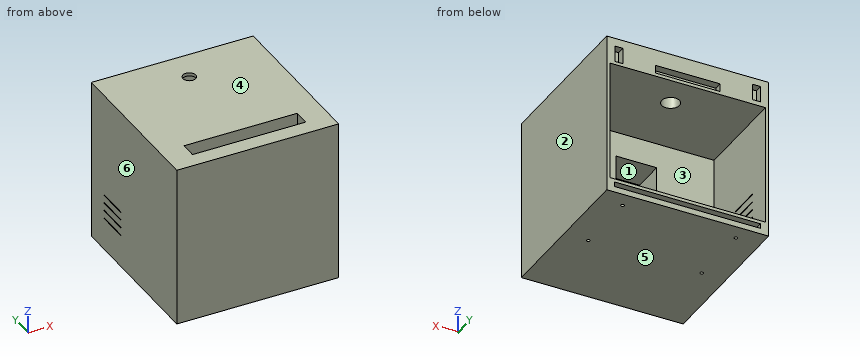
from build123d import *

# Parameters (mm, degrees)
SKETCH1_W           = 100
SKETCH1_H           = 100
BOSS_EXTRUDE1_DEPTH = 100
SKETCH2_W           = 90
SKETCH2_H           = 70
CUT_EXTRUDE1_DEPTH  = 50
SKETCH3_W           = 25
SKETCH3_H           = 25
CUT_EXTRUDE2_DEPTH  = 30
SKETCH4_W           = 70
SKETCH4_H           = 10
CUT_EXTRUDE3_DEPTH  = 70
SKETCH9_W           = 0.5
SKETCH9_H           = 20
CUT_EXTRUDE7_DEPTH  = 10
SKETCH15_W          = 40
SKETCH15_H          = 5
CUT_EXTRUDE8_DEPTH  = 5
SKETCH16_W          = 5
SKETCH16_H          = 10
CUT_EXTRUDE9_DEPTH  = 5
SKETCH17_W          = 5
SKETCH17_H          = 10
CUT_EXTRUDE10_DEPTH = 5
SKETCH20_W          = 70
SKETCH20_H          = 10
CUT_EXTRUDE11_DEPTH = 20
SKETCH21_W          = 90
SKETCH21_H          = 3
CUT_EXTRUDE12_DEPTH = 5
SKETCH23_W          = 90
SKETCH23_H          = 70
CUT_EXTRUDE14_DEPTH = 10
SKETCH26_R          = 1
CUT_EXTRUDE16_DEPTH = 10
SKETCH29_R          = 4
CUT_EXTRUDE20_DEPTH = 11
CUT_EXTRUDE21_START = -2
SKETCH30_R          = 5.5
CUT_EXTRUDE21_DEPTH = 20
SKETCH31_W          = 96
SKETCH31_H          = 74.5
CUT_EXTRUDE22_DEPTH = 60


with BuildPart() as part:
    # Sketch1 → Boss-Extrude1 (new body)
    with BuildSketch(Plane.XY):
        with Locations((50, -50)):
            Rectangle(SKETCH1_W, SKETCH1_H)
    extrude(amount=BOSS_EXTRUDE1_DEPTH)

    # Sketch2 → Cut-Extrude1 (cut)
    with BuildSketch(Plane(origin=(0, 0, 0), x_dir=(1, 0, 0), z_dir=(0, 1, 0))):
        with Locations((50, -45)):
            Rectangle(SKETCH2_W, SKETCH2_H)
    extrude(amount=-CUT_EXTRUDE1_DEPTH, mode=Mode.SUBTRACT)

    # Sketch3 → Cut-Extrude2 (cut)
    with BuildSketch(Plane(origin=(0, -50, 0), x_dir=(1, 0, 0), z_dir=(0, 1, 0))):
        with Locations((50, -55)):
            Rectangle(SKETCH3_W, SKETCH3_H)
    extrude(amount=-CUT_EXTRUDE2_DEPTH, mode=Mode.SUBTRACT)

    # Sketch4 → Cut-Extrude3 (cut)
    with BuildSketch(Plane.XY.offset(100)):
        with Locations((50, -85)):
            Rectangle(SKETCH4_W, SKETCH4_H)
    extrude(amount=-CUT_EXTRUDE3_DEPTH, mode=Mode.SUBTRACT)

    # Sketch9 → Cut-Extrude7 (cut)
    with BuildSketch(Plane.ZY):
        with Locations((20.25, -25)):
            Rectangle(SKETCH9_W, SKETCH9_H)
        with Locations((25.25, -25)):
            Rectangle(SKETCH9_W, SKETCH9_H)
        with Locations((30.25, -25)):
            Rectangle(SKETCH9_W, SKETCH9_H)
        with Locations((35.25, -25)):
            Rectangle(SKETCH9_W, SKETCH9_H)
    extrude(amount=-CUT_EXTRUDE7_DEPTH, mode=Mode.SUBTRACT)

    # Sketch15 → Cut-Extrude8 (cut)
    with BuildSketch(Plane(origin=(0, 0, 0), x_dir=(1, 0, 0), z_dir=(0, 1, 0))):
        with Locations((50, -87.5)):
            Rectangle(SKETCH15_W, SKETCH15_H)
    extrude(amount=-CUT_EXTRUDE8_DEPTH, mode=Mode.SUBTRACT)

    # Sketch16 → Cut-Extrude9 (cut)
    with BuildSketch(Plane(origin=(0, 0, 0), x_dir=(1, 0, 0), z_dir=(0, 1, 0))):
        with Locations((7.5, -90.818061544)):
            Rectangle(SKETCH16_W, SKETCH16_H)
    extrude(amount=-CUT_EXTRUDE9_DEPTH, mode=Mode.SUBTRACT)

    # Sketch17 → Cut-Extrude10 (cut)
    with BuildSketch(Plane(origin=(0, 0, 0), x_dir=(1, 0, 0), z_dir=(0, 1, 0))):
        with Locations((92.5, -90)):
            Rectangle(SKETCH17_W, SKETCH17_H)
    extrude(amount=-CUT_EXTRUDE10_DEPTH, mode=Mode.SUBTRACT)

    # Sketch20 → Cut-Extrude11 (cut)
    with BuildSketch(Plane.XY.offset(30)):
        with Locations((50, -85)):
            Rectangle(SKETCH20_W, SKETCH20_H)
    extrude(amount=-CUT_EXTRUDE11_DEPTH, mode=Mode.SUBTRACT)

    # Sketch21 → Cut-Extrude12 (cut)
    with BuildSketch(Plane(origin=(0, 0, 0), x_dir=(1, 0, 0), z_dir=(0, 1, 0))):
        with Locations((50.175260559, -5)):
            Rectangle(SKETCH21_W, SKETCH21_H)
    extrude(amount=-CUT_EXTRUDE12_DEPTH, mode=Mode.SUBTRACT)

    # Sketch23 → Cut-Extrude14 (cut)
    with BuildSketch(Plane(origin=(0, -50, 0), x_dir=(1, 0, 0), z_dir=(0, 1, 0))):
        with Locations((50, -45)):
            Rectangle(SKETCH23_W, SKETCH23_H)
    extrude(amount=-CUT_EXTRUDE14_DEPTH, mode=Mode.SUBTRACT)

    # Sketch26 → Cut-Extrude16 (cut)
    with BuildSketch(Plane.XY.offset(10)):
        with Locations((15, -10)):
            Circle(SKETCH26_R)
        with Locations((85, -10)):
            Circle(SKETCH26_R)
        with Locations((85, -50)):
            Circle(SKETCH26_R)
        with Locations((15, -50)):
            Circle(SKETCH26_R)
    extrude(amount=-CUT_EXTRUDE16_DEPTH, mode=Mode.SUBTRACT)

    # Sketch29 → Cut-Extrude20 (cut)
    with BuildSketch(Plane.XY.offset(100)):
        with Locations((50, -20)):
            Circle(SKETCH29_R)
    extrude(amount=-CUT_EXTRUDE20_DEPTH, mode=Mode.SUBTRACT)

    # Sketch30 → Cut-Extrude21 (cut)
    with BuildSketch(Plane.XY.offset(100).offset(CUT_EXTRUDE21_START)):
        with Locations((50, -20)):
            Circle(SKETCH30_R)
    extrude(amount=-CUT_EXTRUDE21_DEPTH, mode=Mode.SUBTRACT)

    # Sketch31 → Cut-Extrude22 (cut)
    with BuildSketch(Plane(origin=(0, 0, 0), x_dir=(1, 0, 0), z_dir=(0, 1, 0))):
        with Locations((50, -45.75)):
            Rectangle(SKETCH31_W, SKETCH31_H)
    extrude(amount=-CUT_EXTRUDE22_DEPTH, mode=Mode.SUBTRACT)


solid = part.part
Geometry check sheet. Reference: the model listing, model coordinates, mm. Face numbers are marked on the shaded views. A direction names the side the tool comes from. Give positions to 0.01 mm unless a question says otherwise; leave off trailing zeros. Write each loop counter-clockwise with the first axis right and the second up, starting at its lowest first coordinate (ties: lowest second). Pieces come first, ordered by that corner, then holes. Notation, with made-up numbers: M 71.25,-7 L 104.25,-7 A17 ccw 104.25,23 Z; hole C 26.25,60 d7. An arc over 180 degrees is marked long. Answer as CSV lines item,"result". Start each with the question number.
Q1. Release check for a two-part mould opening along Z. For the marked faces 3, 4, 5 and 6 record: pulls with the +Z half, pulls with the -Z half, needs draft (parallel to the pull), parting line crosses it, or undercut.
Q2. Tool access check on the marked faces 1 and 2. Record the directions out of +Z, -Z, +X, -X, +Y, -Y that give a thin tool (end or side, any length) a straight path to the whole face; none if there is none.
Q3. Go/stop test with a flat-tipped pin: pin 1 (4 mm diameter, centred on x = 61, z = 56.5, fed in from +Y). Record where the tip stops, or that it passes through.
Q4. Material ranges on L1, parallel to Z at x = 18, y = -4; L2, parallel to Y at x = 85, z = 4; L3, parallel to Y at x = 85, z = 7, recorded low to high.
Q5. Section check C-C, the plane z = 12. Record the cut outline in (x, y), then the cut area to 3 significant figures.
Q6. Section check B-B, the plane y = -75.5. Record the cut outline in (x, z).
Q7. Section check A-A, the plane x = 50. Give the number of separate pieces and of enclosed holes in the cut face, then the cut area to 3 significant figures.
Geometry says:
1,face 3,"undercut"
1,face 4,"pulls with the +Z half"
1,face 5,"pulls with the -Z half"
1,face 6,"needs draft"
2,face 1,"+Y"
2,face 2,"+Z, -Z, +X, +Y, -Y"
3,pin 1,"y = -60"
4,L1,"0 to 3.5, 6.5 to 8.5, 83 to 100"
4,L2,"-100 to -51, -49 to -11, -9 to -5"
4,L3,"-100 to -51, -49 to -11, -9 to 0"
5,outline,"M 0,-100 L 100,-100 L 100,0 L 98,0 L 98,-60 L 2,-60 L 2,0 L 0,0 Z; hole M 15,-90 L 85,-90 L 85,-80 L 15,-80 Z"
5,area,"3,540 mm^2"
6,outline,"M 0,0 L 100,0 L 100,100 L 0,100 Z; hole M 37.5,42.5 L 62.5,42.5 L 62.5,67.5 L 37.5,67.5 Z"
7,separate pieces,"3"
7,enclosed holes,"0"
7,area,"3,910 mm^2"
